```python
from build123d import *

# Parameters (mm, degrees)
SKETCH1_R           = 1.5
BOSS_EXTRUDE1_DEPTH = 1.35
CHAMFER1_SIZE       = 0.4


with BuildPart() as part:
    # Sketch1 → Boss-Extrude1 (new, symmetric)
    with BuildSketch(Plane(origin=(0, 0, 0), x_dir=(1, 0, 0), z_dir=(0, 1, 0))):
        with BuildLine():
            Line((-13, 3.5), (13, 3.5))
            ThreePointArc((13, 3.5), (16.5, 0), (13, -3.5))
            Line((13, -3.5), (-13, -3.5))
            ThreePointArc((-13, -3.5), (-16.5, 0), (-13, 3.5))
        make_face()
        with Locations(Location((-13, 0, 0), (0, 0, 90))):
            Circle(SKETCH1_R, mode=Mode.SUBTRACT)
        with Locations(Location((13, 0, 0), (0, 0, 90))):
            Circle(SKETCH1_R, mode=Mode.SUBTRACT)
        with Locations(Location((0, 0, 0), (0, 0, 90))):
            Circle(SKETCH1_R, mode=Mode.SUBTRACT)
    extrude(amount=BOSS_EXTRUDE1_DEPTH, both=True)

    # Chamfer1
    chamfer1_edges = [part.edges().sort_by_distance(p)[0] for p in [
        (16.5, 1.35, 0),
        (0, 1.35, -3.5),
        (-16.5, 1.35, 0),
        (0, 1.35, 3.5),
    ]]
    chamfer(chamfer1_edges, length=CHAMFER1_SIZE)


solid = part.part
```
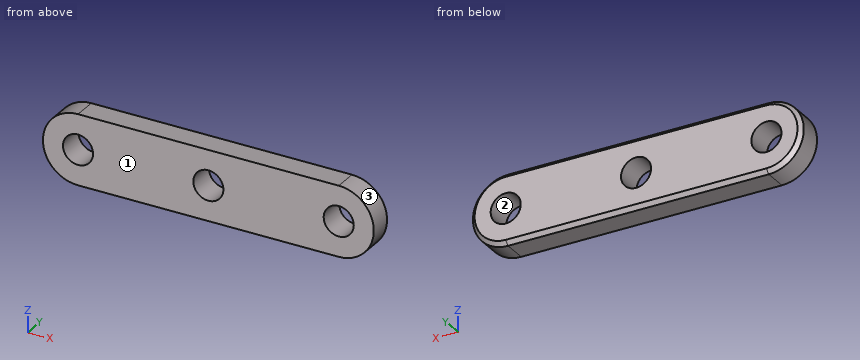
The listing builds one solid part. Answer for the finished solid, in the listing's coordinates (mm). Face numbers are marked on the shaded views. Round coordinates to 2 decimals unless told otherwise and drop trailing zeros. Loops run counter-clockwise (first coordinate to the right, second up) from the corner with the lowest first, then second, coordinate; pieces in that order, holes last. Notation, with made-up numbers: (-17.75, 74) - (9.25, 74) arc R34 cw to (9.25, 110) - close; hole circle Ø10 at (38, 60.25). An arc over 180 degrees is marked (long way). Use one line per item in the form item = value. Start each with the question number.
1. For a pull along X with two mould halves and no side action, classify the marked faces 1, 2 and 3 as pulls with the +X half, pulls with the -X half, needs draft (parallel to the pull), parting line crosses it, or undercut.
2. Consider line 1 (X direction, y = -0.45, z = 0); line 2 (Z direction, x = -13, y = -1.05); line 3 (X direction, y = -0.1, z = -2.5). Determine where each line is inside the solid, lowest interval first. Write a range as [from, to].
3. The part is cut by section C-C on y = 0.55. Determine the outline of the cut face in (x, z).
4. The part is cut by section A-A on x = 0. Determine the outline of the cut face in (y, z), then the cut area to 3 significant figures.
5. The part is cut by section B-B on z = 0. Determine the outline of the cut face in (x, y).
6. Given pin 1 Ø1.8 at (x, z) = (-13, 0) entering from +Y, flat-ended and moving along its own axis, determine where the tip first touches the part or whether it passes through.
Geometry check:
q1.face_1 = needs draft
q1.face_2 = undercut
q1.face_3 = pulls with the +X half
q2.line_1 = [-16.5, -14.5], [-11.5, -1.5], [1.5, 11.5], [14.5, 16.5]
q2.line_2 = [-3.5, -1.5], [1.5, 3.5]
q2.line_3 = [-15.45, 15.45]
q3.outline = (-13, -3.5) - (13, -3.5) arc R3.5 ccw to (13, 3.5) - (-13, 3.5) arc R3.5 ccw to start; hole circle Ø3 at (-13, 0); hole circle Ø3 at (0, 0); hole circle Ø3 at (13, 0)
q4.outline = (-1.35, -3.5) - (0.95, -3.5) - (1.35, -3.1) - (1.35, -1.5) - (-1.35, -1.5) - close; (-1.35, 1.5) - (1.35, 1.5) - (1.35, 3.1) - (0.95, 3.5) - (-1.35, 3.5) - close
q4.area = 10.6 mm^2
q5.outline = (-16.5, -1.35) - (-14.5, -1.35) - (-14.5, 1.35) - (-16.1, 1.35) - (-16.5, 0.95) - close; (-11.5, -1.35) - (-1.5, -1.35) - (-1.5, 1.35) - (-11.5, 1.35) - close; (1.5, -1.35) - (11.5, -1.35) - (11.5, 1.35) - (1.5, 1.35) - close; (14.5, -1.35) - (16.5, -1.35) - (16.5, 0.95) - (16.1, 1.35) - (14.5, 1.35) - close
q6.pin_1 = through
